from build123d import *

# Parameters (mm, degrees)
SKETCH_1_R               = 0.85
EXTRUDE_1_DEPTH          = 3.75
SKETCH_2_W               = 3.1
SKETCH_2_H               = 7.782870542
SKETCH_2_H_2             = 7
CUT_EXTRUDE_1_DEPTH      = 3.25
CUT_EXTRUDE_1_DEPTH_BACK = 3.25
FILLET_1_R               = 1.5
FILLET_2_R               = 0.8
CUT_EXTRUDE_2_DEPTH      = 5.5


with BuildPart() as part:
    # 草图1 → 凸台-拉伸1 (new body, symmetric)
    with BuildSketch(Plane(origin=(0, 0, 0), x_dir=(0, 0, -1), z_dir=(1, 0, 0))):
        Polygon((-2.25, 3.5), (2.25, 3.5), (2.25, -16.5), (-0.659395182, -33), (-2.25, -33), align=None)
        Circle(SKETCH_1_R, mode=Mode.SUBTRACT)
        with Locations((0, -11)):
            Circle(SKETCH_1_R, mode=Mode.SUBTRACT)
    extrude(amount=EXTRUDE_1_DEPTH, both=True)

    # 草图2 → 切除-拉伸1 (cut, two sides)
    with BuildSketch(Plane.XY) as cut_extrude_1_sk:
        with Locations((0, 0.891435271)):
            Rectangle(SKETCH_2_W, SKETCH_2_H)
        with Locations((0, -11)):
            Rectangle(SKETCH_2_W, SKETCH_2_H_2)
    extrude(amount=CUT_EXTRUDE_1_DEPTH, mode=Mode.SUBTRACT)
    extrude(cut_extrude_1_sk.sketch, amount=-CUT_EXTRUDE_1_DEPTH_BACK, mode=Mode.SUBTRACT)

    # 圆角1
    fillet_1_edges = [part.edges().sort_by_distance(p)[0] for p in [
        (-2.65, 3.5, 2.25),
        (-2.65, 3.5, -2.25),
        (2.65, 3.5, 2.25),
        (2.65, 3.5, -2.25),
    ]]
    fillet(fillet_1_edges, radius=FILLET_1_R)

    # 圆角2
    fillet_2_edges = [part.edges().sort_by_distance(p)[0] for p in [
        (-1.55, -3, 0),
        (1.55, -3, 0),
        (-1.55, -7.5, 0),
        (1.55, -7.5, 0),
        (1.55, -14.5, 0),
        (-1.55, -14.5, 0),
    ]]
    fillet(fillet_2_edges, radius=FILLET_2_R)

    # 草图3 → 切除-拉伸2 (cut, through all)
    with BuildSketch(Plane.XY.offset(2.25)):
        Polygon((-3.75, -15), (-2, -33), (-6.857355495, -33), align=None)
        Polygon((6.857355495, -33), (3.75, -15), (2, -33), align=None)
    extrude(amount=-CUT_EXTRUDE_2_DEPTH, mode=Mode.SUBTRACT)


solid = part.part
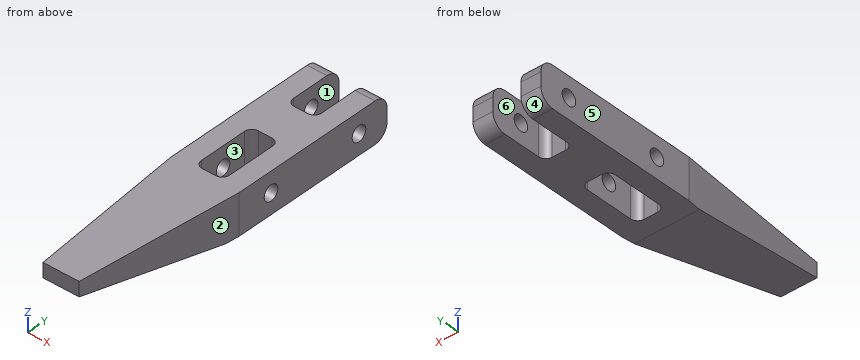
Here's how the part is built. I have some questions about the finished solid (model axes, mm). Face numbers are marked on the shaded views. A direction names the side the tool comes from. Round coordinates to 2 decimals unless told otherwise and drop trailing zeros. Loops run counter-clockwise (first coordinate to the right, second up) from the corner with the lowest first, then second, coordinate; pieces in that order, holes last.
1. For P1, Ø1.2, axis at x = 0, z = -0.5, coming from the +Y side; P2, Ø1, axis at y = -11, z = 0, coming from the -X side; P3, Ø1.5, axis at y = -16, z = -1, coming from the -X side, each with a flat end and sliding along its axis, tell me the tip position at first contact or that it passes through.
Answer list:
P1: stops at y = -3
P2: passes through
P3: stops at x = -3.73
2. If we section it at A-A on y = -11: Write out the boundary of the cut face in (x, z), plus the area to 3 significant figures.
Answer list:
outline: (-3.75, -2.25) - (-1.55, -2.25) - (-1.55, -0.85) - (-3.75, -0.85) - close; (-3.75, 0.85) - (-1.55, 0.85) - (-1.55, 2.25) - (-3.75, 2.25) - close; (1.55, -2.25) - (3.75, -2.25) - (3.75, -0.85) - (1.55, -0.85) - close; (1.55, 0.85) - (3.75, 0.85) - (3.75, 2.25) - (1.55, 2.25) - close
area: 12.3 mm2
3. If we section it at B-B on x = 3.25: Write out the boundary of the cut face in (y, z).
Answer list:
outline: (-20.14, -1.61) - (-16.5, -2.25) - (2, -2.25) arc R1.5 ccw to (3.5, -0.75) - (3.5, 0.75) arc R1.5 ccw to (2, 2.25) - (-20.14, 2.25) - close; hole circle Ø1.7 at (-11, 0); hole circle Ø1.7 at (0, 0)
4. If we section it at D-D on z = 0.25: Count the separate pieces of the cut face and the enclosed holes in it, plus the area to 3 significant figures.
Answer list:
separate pieces: 4
enclosed holes: 0
area: 177 mm2
5. If I drill on line 1 along X through (y, z) = (-13, 1.95); line 2 along Z through (x, y) = (-2.15, -11); line 3 along X through (y, z) = (-16.5, -0.2), over which ranges is the centre line in solid material (lowest first)?
Answer list:
line 1: x = -3.75 to -1.55, 1.55 to 3.75
line 2: z = -2.25 to -0.85, 0.85 to 2.25
line 3: x = -3.6 to 3.6
6. If we section it at C-C on z = -1.3: Write out the boundary of the cut face in (x, y), plus the area to 3 significant figures.
Answer list:
outline: (-3.75, -15) - (-3.08, -21.89) - (3.08, -21.89) - (3.75, -15) - (3.75, 3.4) - (1.55, 3.4) - (1.55, -2.2) arc R0.8 cw to (0.75, -3) - (-0.75, -3) arc R0.8 cw to (-1.55, -2.2) - (-1.55, 3.4) - (-3.75, 3.4) - close; hole (-1.55, -13.7) arc R0.8 ccw to (-0.75, -14.5) - (0.75, -14.5) arc R0.8 ccw to (1.55, -13.7) - (1.55, -8.3) arc R0.8 ccw to (0.75, -7.5) - (-0.75, -7.5) arc R0.8 ccw to (-1.55, -8.3) - close
area: 144 mm2
7. Which directions (+Z, -Z, +X, -X, +Y, -Y) give clear straight access to the entire face, cutting with the end or side of a thin tool? Please do the marked faces 1, 2 and 3.
Answer list:
face 1: +Z, -Z, +Y
face 2: +Z, -Z, +X, -Y
face 3: +Z, -Z
8. We'd pull the mould along X, two halves only. Please class the marked faces 4, 5 and 6: +X half, -X half, draft (parallel to the pull), parting line (faces both ways), or undercut.
Answer list:
face 4: draft
face 5: -X half
face 6: undercut
